Autodesk Inventor part; units mm, degrees
ref_plane "YZ Plane" through (0, 0, 0) normal (1, 0, 0) x (0, 1, 0)
ref_plane "XZ Plane" through (0, 0, 0) normal (0, 1, 0) x (-1, 0, 0)
ref_plane "XY Plane" through (0, 0, 0) normal (0, 0, 1) x (1, 0, 0)
ref_plane "Work Plane1" through (0, 0, 0) normal (0, 0, 1) x (1, 0, 0)
sketch "Sketch1" plane through (0, 0, 0) normal (0, 0, 1) x (1, 0, 0)
  arc A0 (12.5, 11.5) -> (11.5, 12.5) centre (11.5, 11.5) ccw
  line L0 (8.5, 12.5) -> (11.5, 12.5)
  arc A1 (8.5, 12.5) -> (7.5, 11.5) centre (8.5, 11.5) ccw
  line L1 (7.5, 1.5) -> (7.5, 11.5)
  arc A2 (-12.5, -11.5) -> (-11.5, -12.5) centre (-11.5, -11.5) ccw
  line L2 (7.5, -12.5) -> (-11.5, -12.5)
  arc A3 (7.5, -12.5) -> (12.5, -7.5) centre (7.5, -7.5) ccw
  line L3 (12.5, 11.5) -> (12.5, -7.5)
  arc A4 (-11.5, 1.5) -> (-12.5, 0.5) centre (-11.5, 0.5) ccw
  line L4 (-12.5, 0.5) -> (-12.5, -11.5)
  line L5 (7.5, 1.5) -> (-11.5, 1.5)
  circle A5 centre (-2.5, -3) radius 1.65
  arc A6 (12.5, 11.5) -> (11.5, 12.5) centre (11.5, 11.5) ccw
  line L6 (12.5, -7.5) -> (12.5, 11.5)
  arc A7 (7.5, -12.5) -> (12.5, -7.5) centre (7.5, -7.5) ccw
  line L7 (1.0011, -12.5) -> (7.5, -12.5)
  line L8 (-6.0011, -12.5) -> (1.0011, -12.5)
  line L9 (-11.5, -12.5) -> (-6.0011, -12.5)
  arc A8 (-12.5, -11.5) -> (-11.5, -12.5) centre (-11.5, -11.5) ccw
  line L10 (-12.5, -8.5) -> (-12.5, -11.5)
  arc A9 (-11.5, -7.5) -> (-12.5, -8.5) centre (-11.5, -8.5) ccw
  line L11 (2.5, -7.5) -> (-11.5, -7.5)
  arc A10 (2.5, -7.5) -> (7.5, -2.5) centre (2.5, -2.5) ccw
  line L12 (7.5, 11.5) -> (7.5, -2.5)
  arc A11 (8.5, 12.5) -> (7.5, 11.5) centre (8.5, 11.5) ccw
  line L13 (8.5, 12.5) -> (11.5, 12.5)
revolve "Revolution1" add sketch "Sketch1" angle 90 about axis through (8.5, 12.5, 0) along (-1, 0, 0) contours L3 A3 L2 A2 L4 A9 L11 A10 L12 L1 A1 L0 A0
sketch "Sketch2" plane through (8.5, 12.5, 0) normal (0, 1, 0) x (1, 0, 0)
  line L0 (4, -20) -> (4, -1)
  arc A0 (4, -1) -> (3, 0) centre (3, -1) ccw
  line L1 (3, 0) -> (0, 0)
  arc A1 (0, 0) -> (-1, -1) centre (0, -1) ccw
  line L2 (-1, -1) -> (-1, -15)
  arc A2 (-21, -24) -> (-20, -25) centre (-20, -24) ccw
  line L3 (-20, -25) -> (-1, -25)
  arc A3 (-1, -25) -> (4, -20) centre (-1, -20) ccw
  line L4 (-21, -21) -> (-21, -24)
  line L5 (-6, -20) -> (-20, -20)
  arc A4 (-20, -20) -> (-21, -21) centre (-20, -21) ccw
  arc A5 (-6, -20) -> (-1, -15) centre (-6, -15) ccw
  point P0 (-8.5, 0)
extrude "Extrusion1" add sketch "Sketch2" along normal up to surface (79.8139 mm away)
sketch "Sketch5" plane through (7.5, -12.5, 0) normal (0, 0, -1) x (-1, 0, 0)
  line L0 (20, 99.8139) -> (-1, 99.8139)
  line L1 (-1, 99.8139) -> (-1, 94.8139)
  line L2 (-1, 94.8139) -> (20, 94.8139)
  line L3 (20, 94.8139) -> (20, 99.8139)
  line L4 (20, 25) -> (20, 104.8139)
  line L5 (19, 104.8139) -> (5, 104.8139)
  point P0 (7.5, 12.5)
  point P1 (-1, 104.8139)
  dimension "d10" = 5
  dimension "d11" = 5
extrude "Extrusion4" add sketch "Sketch5" against normal up to next
sketch "Sketch6" plane through (-12.5, 82.3139, 0) normal (0, -1, 0) x (1, 0, 0)
  circle A0 centre (13.75, 10) radius 1.65
  circle A1 centre (6.25, 10) radius 1.65
  line L0 (13.75, 10) -> (6.25, 10) construction
  line L1 (20, 15) -> (20, 1)
  line L2 (20, 2.0913) -> (0, 2.0913) construction
  line L3 (21, 0) -> (0, 0)
  line L4 (10, 0) -> (10, 20) construction
  line L5 (1, 20) -> (15, 20)
  line L6 (0, 0) -> (0, 21)
  point P0 (12.5, 0)
  point P1 (10, 2.0913)
  point P2 (10, 10)
  point P3 (20, 11)
  point P4 (0, 12)
  dimension "d14" = 7.5
  dimension "d15" = 3.3
extrude "Extrusion5" cut sketch "Sketch6" against normal through all
sketch "Sketch8" plane through (7.5, -12.5, 0) normal (0, 0, -1) x (-1, 0, 0)
  arc A0 (20, 4) -> (19, 5) centre (19, 4) ccw
  line L0 (-1, 25) -> (-1, 94.8139)
  line L1 (20, 4) -> (-1, 4)
  line L2 (-1, 4) -> (-1, 14)
  line L3 (-1, 14) -> (20, 14)
  line L4 (20, 14) -> (20, 4)
  point P0 (7.5, 12.5)
  dimension "d18" = 10
extrude "Extrusion6" add sketch "Sketch8" against normal up to next
sketch "Sketch9" plane through (7.5, -12.5, 0) normal (0, 0, -1) x (-1, 0, 0)
  circle A0 centre (10, 9.5) radius 1.65
  arc A1 (-4, 25) -> (-5, 24) centre (-4, 24) ccw
  line L0 (-1, 25) -> (-4, 25)
  arc A2 (0, 24) -> (-1, 25) centre (-1, 24) ccw
  line L1 (0, 14) -> (0, 24)
  arc A3 (19, 0) -> (20, 1) centre (19, 1) ccw
  line L2 (0, 0) -> (19, 0)
  arc A4 (-5, 5) -> (0, 0) centre (0, 5) ccw
  line L3 (-5, 24) -> (-5, 5)
  line L4 (20, 1) -> (20, 14)
  line L5 (20, 9.5) -> (0, 9.5) construction
  line L6 (10, 5) -> (10, 14) construction
  line L7 (20, 14) -> (0, 14)
  arc A5 (20, 13) -> (19, 14) centre (19, 13) ccw
  line L8 (20, 13) -> (20, 1)
  line L9 (0, 14) -> (19, 14)
  circle A6 centre (10, 9.5) radius 1.65
  point P0 (7.5, 12.5)
  point P1 (20, 4)
  point P2 (10, 9.5)
  dimension "d21" = 3.3
extrude "Extrusion7" cut sketch "Sketch9" against normal blind 10 contours A0
sketch "Sketch11" plane through (-2.5, -3, 10) normal (0, 0, -1) x (-1, 0, 0)
  line L0 (0, -3.3486) -> (-2.9, -1.6743)
  line L1 (-2.9, -1.6743) -> (-2.9, 1.6743)
  line L2 (-2.9, 1.6743) -> (0, 3.3486)
  line L3 (0, 3.3486) -> (2.9, 1.6743)
  line L4 (2.9, 1.6743) -> (2.9, -1.6743)
  line L5 (2.9, -1.6743) -> (0, -3.3486)
  line L6 (0, 6.2514) -> (0, -6.2514) construction
  circle A0 centre (0, 0) radius 1.65 construction
  circle A1 centre (0, 0) radius 1.65
  point P0 (-2.5, 3)
  dimension "d27" = 9.6
  dimension "d28" = 5.8
extrude "Extrusion8" cut sketch "Sketch11" along normal blind 2.7
sketch "Sketch12" plane through (-12.5, 1.5, 0) normal (0, 1, 0) x (1, 0, 0)
  line L0 (7.1, -10) -> (10, -10)
  line L1 (10, -10) -> (12.9, -10)
  line L2 (12.9, -10) -> (10, -10)
  line L3 (10, -10) -> (7.1, -10)
  line L4 (7.1, -10) -> (7.1, -7.3)
  line L5 (7.1, -10) -> (7.1, -7.3)
  line L6 (7.1, -7.3) -> (12.9, -7.3)
  line L7 (12.9, -10) -> (12.9, -7.3)
  line L8 (12.9, -7.3) -> (12.9, -10)
  point P0 (12.5, 0)
  dimension "d31" = 2.7
extrude "Extrusion9" cut sketch "Sketch12" against normal up to next
sketch "Sketch13" plane through (7.5, -12.5, 10) normal (0, 0, -1) x (-1, 0, 0)
  circle A0 centre (10, 9.5) radius 1.65
  circle A1 centre (10, 9.5) radius 1.65
  point P0 (7.5, 12.5)
extrude "Extrusion10" cut sketch "Sketch13" against normal blind 5
properties part number "frame-foot"
Part model, mm, in its own coordinate system. A direction names the side the tool comes from. Give positions to 0.01 mm unless a question says otherwise; leave off trailing zeros. Order: outer loops, then holes, each group sorted by start corner. A loop starts at its lowest first (then second) coordinate and runs counter-clockwise, first axis right, second up. Notation, with made-up numbers: (59, -26) - (108, -26) arc R16 cw to (108, -2) - close; hole circle Ø11 at (27.5, -2.75). An arc over 180 degrees is marked (long way). Use one line per item in the form item = value.
Item 1: Pin check, flat tips, straight feed: pin 1 Ø2 at (x, y) = (-2.5, -3) entering from +Z; pin 2 Ø1.5 at (y, z) = (81, 4) entering from -X; pin 3 Ø4.5 at (x, z) = (1.25, 10) entering from +Y. Stop position of each tip, or through.
Solution:
pin_1 = 20.37
pin_2 = 7.5
pin_3 = 87.31
Item 2: Two-plate mould, pull along Y, no slides. Class faces 6 (the face through (5, 92.314, 21)), 7 (the face through (-2, 52, 25)), 8 (the face through (-5.4, -2, 9)): released by +Y, released by -Y, zero draft, split by the parting line, or undercut.
Solution:
face_6 = released by +Y
face_7 = zero draft
face_8 = undercut
Item 3: Probe probe 1 along Z at (x, y) = (1.25, 85.8); probe 2 along Y at (x, z) = (-2.5, 3.75); probe 3 along X at (y, z) = (41, 3.25). List the from-to ranges inside material, lowest first. Write a range as from..to.
Solution:
probe_1 = 0..8.35, 11.65..25
probe_2 = -12.22..-4.65, -1.35..1.5, 82.31..87.31
probe_3 = 7.5..12.5
Item 4: Slice it at A-A on x = -10. Give the cut face in (y, z).
Solution:
outline = (-12.5, 0) - (1.5, 0) - (1.5, 16.7) arc R20 cw to (12.5, 20) - (82.31, 20) - (82.31, 0) - (87.31, 0) - (87.31, 20) - (92.31, 20) - (92.31, 25) - (12.5, 25) arc R25 ccw to start
Item 5: Which spindle directions (+Z, -Z, +X, -X, +Y, -Y) get a long thin tool onto all of the face, cutting with end or side? Do faces 1 (the face through (6.07, 89.78, 18.5)), 2 (the face through (-1.19, -4, 3.6)), 3 (the face through (0.4, -2, 9)), 4 (the face through (-7.56, 84.78, 9)), 5 (the face through (-4.598, 6.68, 19.135)). Say none if no direction does.
Solution:
face_1 = -Z, -X, +Y
face_2 = -Z
face_3 = none
face_4 = +Y
face_5 = -Z, -X
Item 6: Slice it at C-C on x = 10.25. Give the cut face in (y, z), and give its area (3 significant figures).
Solution:
outline = (-11.68, 0) - (92.31, 0) - (92.31, 24.18) - (12.5, 24.18) arc R24.18 ccw to start
area = 2,390 mm2
Item 7: Slice it at B-B on y = 60. Give the cut face in (x, z).
Solution:
outline = (-12.5, 21) arc R1 ccw to (-11.5, 20) - (2.5, 20) arc R5 cw to (7.5, 15) - (7.5, 1) arc R1 ccw to (8.5, 0) - (11.5, 0) arc R1 ccw to (12.5, 1) - (12.5, 20) arc R5 ccw to (7.5, 25) - (-11.5, 25) arc R1 ccw to (-12.5, 24) - close
